For this review, use the dimensioned drawing (mm, ordinates from the lowest corner) and the shaded views. A direction names the side the tool comes from. Coordinates: 2 decimals unless noted, no trailing zeros. Loops run counter-clockwise (first coordinate to the right, second up) from the corner with the lowest first, then second, coordinate; pieces in that order, holes last. Notation, with made-up numbers: M 89.5,-40 L 111.5,-40 A19 ccw 111.5,-9 Z; hole C -9,-7.75 d3. An arc over 180 degrees is marked long. One line per item, written item: value.
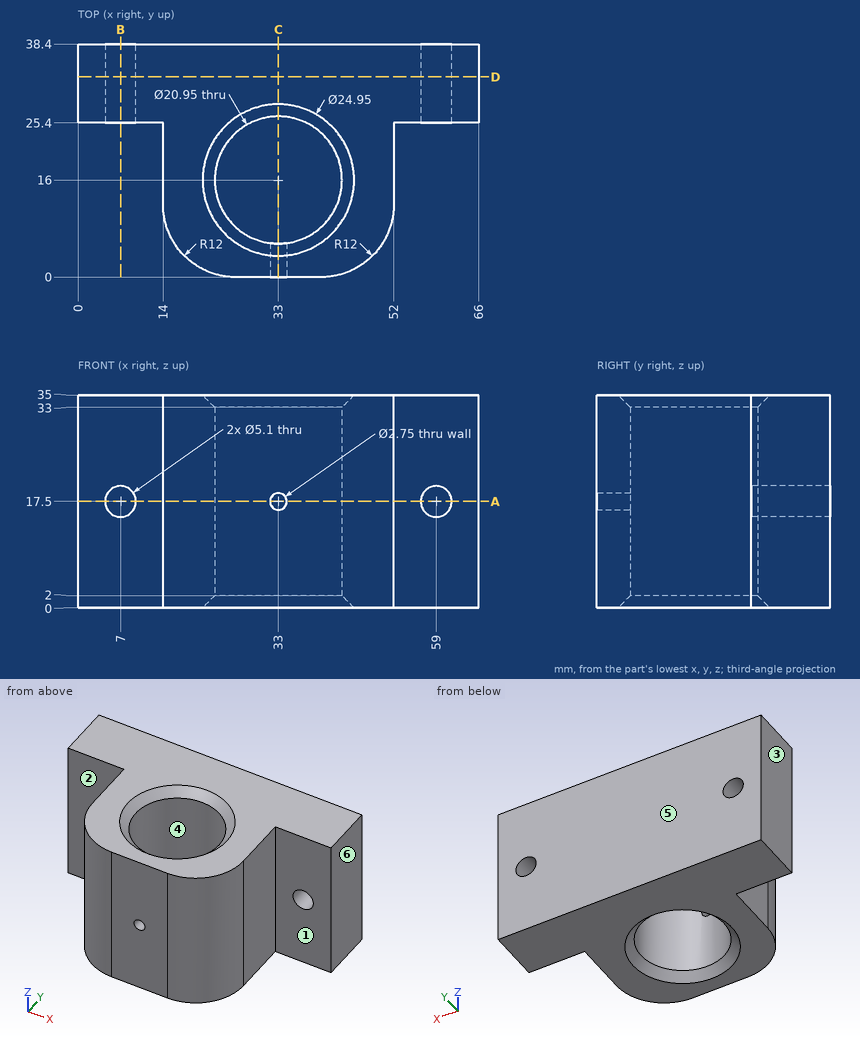
(1) Tool access review of the marked faces 1, 2 and 3: name each direction out of +Z, -Z, +X, -X, +Y, -Y from which nothing blocks a thin tool from reaching the whole face with its end or side.
Reply:
face 1: +Z, -Z, +X, -Y
face 2: +Z, -Z, -X, -Y
face 3: +Z, -Z, -X, +Y, -Y
(2) We need section C-C on x = 33. State the section outline as (y, z) points (3 decimals), then the cut area to 3 significant figures.
Reply:
outline: M 0,0 L 3.525,0 L 5.525,2 L 5.525,16.125 L 0,16.125 Z; M 0,18.875 L 5.525,18.875 L 5.525,33 L 3.525,35 L 0,35 Z; M 26.475,2 L 28.475,0 L 38.4,0 L 38.4,35 L 28.475,35 L 26.475,33 Z
area: 588 mm2
(3) To check wall thickness, follow line 1 along Y through (x, z) = (33, 15.5) (3 decimals); line 2 along Z through (x, y) = (59, 33); line 3 along Y through (x, z) = (61.5, 13). State the ranges of each line that lie inside material, in increasing order. Write a range as [from, to].
Reply:
line 1: y = [0, 5.525], [26.475, 38.4]
line 2: z = [0, 14.95], [20.05, 35]
line 3: y = [25.4, 38.4]
(4) Insertion check: pin 1 (12 mm diameter, centred on x = 8, y = 21, fed in from -Z); pin 2 (7 mm diameter, centred on x = 7, z = 13.5, fed in from -Y); pin 3 (8 mm diameter, centred on y = 8.5, z = 25, fed in from -X); pin 4 (1.5 mm diameter, centred on x = 24.5, z = 29, fed in from -Y). Each pin has a flat end and moves straight along its axis. Give the tip position at first contact, or say it passes through.
Reply:
pin 1: stops at z = 0
pin 2: stops at y = 25.4
pin 3: stops at x = 14
pin 4: stops at y = 0.02
(5) We need section A-A on z = 17.5. State the section outline as (x, y) points (3 decimals).
Reply:
outline: M 0,25.4 L 4.45,25.4 L 4.45,38.4 L 0,38.4 Z; M 9.55,25.4 L 14,25.4 L 14,12 A12 ccw 26,0 L 31.625,0 L 31.625,5.616 A10.475 cw long 34.375,5.616 L 34.375,0 L 40,0 A12 ccw 52,12 L 52,25.4 L 56.45,25.4 L 56.45,38.4 L 9.55,38.4 Z; M 61.55,25.4 L 66,25.4 L 66,38.4 L 61.55,38.4 Z
(6) Mouldability with a two-part tool opening along X and no side actions: class the marked faces 4, 5 and 6 as released by +X, released by -X, zero draft, split by the parting line, or undercut.
Reply:
face 4: undercut
face 5: zero draft
face 6: released by +X
(7) We need section B-B on x = 7. State the section outline as (y, z) points.
Reply:
outline: M 25.4,0 L 38.4,0 L 38.4,14.95 L 25.4,14.95 Z; M 25.4,20.05 L 38.4,20.05 L 38.4,35 L 25.4,35 Z
(8) We need section D-D on y = 33. State the section outline as (x, z) points.
Reply:
outline: M 0,0 L 66,0 L 66,35 L 0,35 Z; hole C 7,17.5 d5.1; hole C 59,17.5 d5.1
